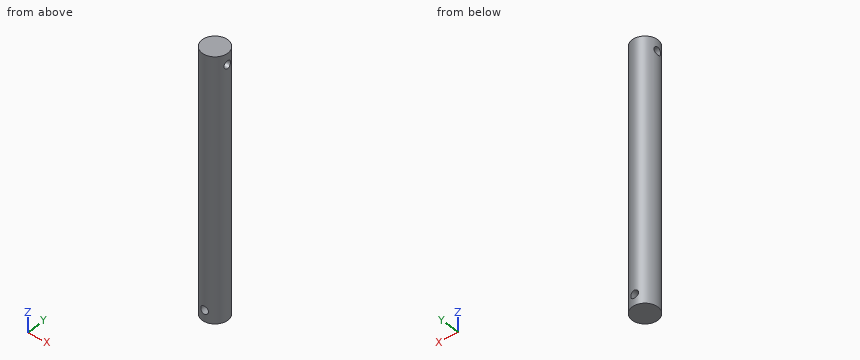
from build123d import *

# Parameters (mm, degrees)
SKETCH3_R           = 5.75
BOSS_EXTRUDE1_DEPTH = 117.15
SKETCH4_R           = 1.75
CUT_EXTRUDE2_DEPTH  = 15
SKETCH5_R           = 1.75
CUT_EXTRUDE3_DEPTH  = 15


with BuildPart() as part:
    # Sketch3 → Boss-Extrude1 (new body)
    with BuildSketch(Plane.XY):
        Circle(SKETCH3_R)
    extrude(amount=BOSS_EXTRUDE1_DEPTH)

    # Sketch4 → Cut-Extrude2 (cut, symmetric)
    with BuildSketch(Plane(origin=(0, 0, 0), x_dir=(1, 0, 0), z_dir=(0, 1, 0))):
        with Locations(Location((0, -5, 0), (0, 0, 90))):
            Circle(SKETCH4_R)
    extrude(amount=CUT_EXTRUDE2_DEPTH, both=True, mode=Mode.SUBTRACT)

    # Sketch5 → Cut-Extrude3 (cut, symmetric)
    with BuildSketch(Plane(origin=(0, 0, 0), x_dir=(0, 0, -1), z_dir=(1, 0, 0))):
        with Locations(Location((-112.15, 0, 0), (0, 0, 179.999999999))):
            Circle(SKETCH5_R)
    extrude(amount=CUT_EXTRUDE3_DEPTH, both=True, mode=Mode.SUBTRACT)


solid = part.part
Read the model definition and answer for the solid it produces. Units are mm, in the model's axes. Coordinates: 2 decimals unless noted, no trailing zeros. Loops run counter-clockwise (first coordinate to the right, second up) from the corner with the lowest first, then second, coordinate; pieces in that order, holes last. Notation, with made-up numbers: (36, 73) - (76, 73) arc R25 ccw to (76, 111) - close; hole circle Ø2 at (56, -38.5). An arc over 180 degrees is marked (long way). Answer in a Markdown table with one row per item.
Q1. Find section B-B on y = -4. Write down the section's boundary in (x, z), plus the area to 3 significant figures.
Here are the results:
| item | result |
|---|---|
| outline | (-4.13, 0) - (4.13, 0) - (4.13, 117.15) - (-4.13, 117.15) - close; hole circle Ø3.5 at (0, 5) |
| area | 958 mm^2 |
Q2. Find section D-D on z = 112.15. Write down the section's boundary in (x, y), plus the area to 3 significant figures.
Here are the results:
| item | result |
|---|---|
| outline | (-5.48, -1.75) arc R5.75 ccw to (5.48, -1.75) - close; (-5.48, 1.75) - (5.48, 1.75) arc R5.75 ccw to start |
| area | 64.2 mm^2 |
Q3. Find section C-C on z = 94. Write down the section's boundary in (x, y).
Here are the results:
| item | result |
|---|---|
| outline | circle Ø11.5 at (0, 0) |
Q4. Find section A-A on x = 0. Write down the section's boundary in (y, z), plus the area to 3 significant figures.
Here are the results:
| item | result |
|---|---|
| outline | (-5.75, 0) - (5.75, 0) - (5.75, 3.25) - (-5.75, 3.25) - close; (-5.75, 6.75) - (5.75, 6.75) - (5.75, 117.15) - (-5.75, 117.15) - close; hole circle Ø3.5 at (0, 112.15) |
| area | 1,300 mm^2 |
Q5. Given P1, Ø2, axis at x = 3, z = 58, coming from the -Y side; P2, Ø5, axis at x = 3, z = 37.5, coming from the -Y side; P3, Ø1, axis at x = -4, z = 39.5, coming from the +Y side, each flat-ended and moving along its own axis, determine where each tip first touches the part or whether it passes through.
Here are the results:
| item | result |
|---|---|
| P1 | stops at y = -5.39 |
| P2 | stops at y = -5.73 |
| P3 | stops at y = 4.56 |
Q6. Straight lines are drawn through the part: line 1 along X through (y, z) = (0, 5); line 2 along Y through (x, z) = (0.75, 112.15); line 3 along Z through (x, y) = (-1, -4.5). For each, find the intervals that lie inside material, in ascending order. Write a range as [from, to].
Here are the results:
| item | result |
|---|---|
| line 1 | x = [-5.75, -1.75], [1.75, 5.75] |
| line 2 | y = [-5.7, -1.75], [1.75, 5.7] |
| line 3 | z = [0, 3.56], [6.44, 117.15] |
